Check sheet for the modelled part. Datum: model origin and axes. Units: mm. Face numbers are marked on the shaded views. A direction names the side the tool comes from. Give positions to 0.01 mm unless a question says otherwise; leave off trailing zeros. Order: outer loops, then holes, each group sorted by start corner. A loop starts at its lowest first (then second) coordinate and runs counter-clockwise, first axis right, second up.
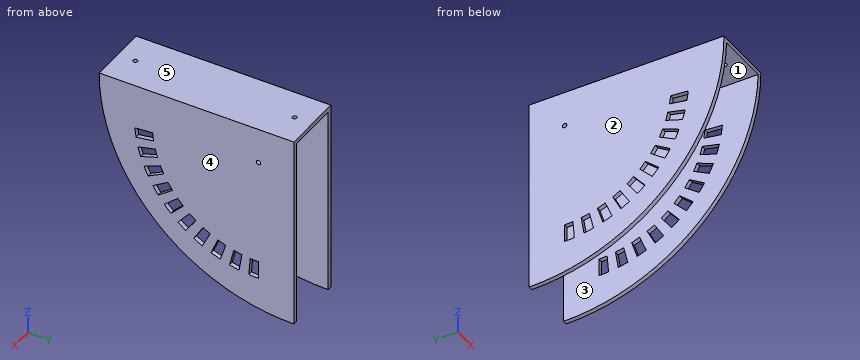
```python
from build123d import *

# Parameters (mm, degrees)
SKETCH1_W             = 5
SKETCH1_H             = 220
BOSS_EXTRUDE1_DEPTH   = 220
BOSS_EXTRUDE1_2_DEPTH = 220
SKETCH2_W             = 60
SKETCH2_H             = 220
BOSS_EXTRUDE2_DEPTH   = 5
CUT_EXTRUDE1_DEPTH    = 110
SKETCH7_R             = 2.5
CUT_EXTRUDE6_DEPTH    = 134
SKETCH9_R             = 2.5
CUT_EXTRUDE8_DEPTH    = 134


with BuildPart() as part:
    # Sketch1 → Boss-Extrude1 (new body)
    with BuildSketch(Plane.XY):
        with Locations((32.5, 0)):
            Rectangle(SKETCH1_W, SKETCH1_H)
    extrude(amount=BOSS_EXTRUDE1_DEPTH)



with BuildPart() as body_2:
    # Sketch1 → Boss-Extrude1 2 (new body)
    with BuildSketch(Plane.XY):
        with Locations((-32.5, 0)):
            Rectangle(SKETCH1_W, SKETCH1_H)
    extrude(amount=BOSS_EXTRUDE1_2_DEPTH)


with BuildPart() as part_1:
    add(part.part)

    add(body_2.part)  # Boss-Extrude2 merges body 2
    # Sketch2 → Boss-Extrude2 (add)
    with BuildSketch(Plane.XY.offset(220)):
        Rectangle(SKETCH2_W, SKETCH2_H)
    extrude(amount=-BOSS_EXTRUDE2_DEPTH)

    # Sketch3 → Cut-Extrude1 (cut)
    with BuildSketch(Plane.ZY.offset(35)):
        with BuildLine():
            Line((0, 110), (0, -110))
            Line((0, -110), (220, -110))
            ThreePointArc((220, -110), (64.436508139, -45.563491861), (0, 110))
        make_face()
    extrude(amount=-CUT_EXTRUDE1_DEPTH, mode=Mode.SUBTRACT)

    # Sketch7 → Cut-Extrude6 (cut)
    with BuildSketch(Plane(origin=(0, 0, 215), x_dir=(-1, 0, 0), z_dir=(0, 0, -1))):
        with Locations((0, 90)):
            Circle(SKETCH7_R)
        with Locations((0, -90)):
            Circle(SKETCH7_R)
    extrude(amount=-CUT_EXTRUDE6_DEPTH, mode=Mode.SUBTRACT)

    # Sketch9 → Cut-Extrude8 (cut)
    with BuildSketch(Plane.ZY.offset(35)):
        with BuildLine():
            ThreePointArc((60.369919952, 60.584908513), (60.092515651, 65.288822109), (60, 70))
            Line((60, 70), (40, 70))
            ThreePointArc((40, 70), (40.107934926, 64.503625794), (40.431573277, 59.015726598))
            Line((40.431573277, 59.015726598), (60.369919952, 60.584908513))
        make_face()
        with BuildLine():
            ThreePointArc((63.315609552, 41.986556337), (62.305766352, 46.589161358), (61.477399129, 51.227864195))
            Line((61.477399129, 51.227864195), (41.723632317, 48.099174894))
            ThreePointArc((41.723632317, 48.099174894), (42.690060744, 42.687354918), (43.868211144, 37.31764906))
            Line((43.868211144, 37.31764906), (63.315609552, 41.986556337))
        make_face()
        with BuildLine():
            ThreePointArc((69.134456099, 24.077988116), (67.417039689, 28.465953151), (65.873218045, 32.917960675))
            Line((65.873218045, 32.917960675), (46.852087719, 26.737620788))
            ThreePointArc((46.852087719, 26.737620788), (48.653212971, 21.543612009), (50.656865448, 16.424319469))
            Line((50.656865448, 16.424319469), (69.134456099, 24.077988116))
        make_face()
        with BuildLine():
            ThreePointArc((77.683180278, 7.300172234), (75.300479151, 11.36545102), (73.079217097, 15.521140031))
            Line((73.079217097, 15.521140031), (55.259086614, 6.441330036))
            ThreePointArc((55.259086614, 6.441330036), (57.85055901, 1.59302619), (60.63037699, -3.14979906))
            Line((60.63037699, -3.14979906), (77.683180278, 7.300172234))
        make_face()
        with BuildLine():
            ThreePointArc((88.751284128, -7.9337658), (85.761968294, -4.291273917), (82.917960675, -0.534230275))
            Line((82.917960675, -0.534230275), (66.737620788, -12.289935321))
            ThreePointArc((66.737620788, -12.289935321), (70.055629677, -16.673152903), (73.543164816, -20.922726766))
            Line((73.543164816, -20.922726766), (88.751284128, -7.9337658))
        make_face()
        with BuildLine():
            ThreePointArc((102.0662342, -21.248715872), (98.543910536, -18.118701132), (95.147186258, -14.852813742))
            Line((95.147186258, -14.852813742), (81.005050634, -28.994949366))
            ThreePointArc((81.005050634, -28.994949366), (84.967895625, -32.805151321), (89.077273234, -36.456835184))
            Line((89.077273234, -36.456835184), (102.0662342, -21.248715872))
        make_face()
        with BuildLine():
            ThreePointArc((117.300172234, -32.316819722), (113.331572038, -29.776353476), (109.465769725, -27.082039325))
            Line((109.465769725, -27.082039325), (97.710064679, -43.262379212))
            ThreePointArc((97.710064679, -43.262379212), (102.220167377, -46.405745722), (106.85020094, -49.36962301))
            Line((106.85020094, -49.36962301), (117.300172234, -32.316819722))
        make_face()
        with BuildLine():
            ThreePointArc((134.077988116, -40.865543901), (129.760831496, -38.977180859), (125.521140031, -36.920782903))
            Line((125.521140031, -36.920782903), (116.441330036, -54.740913386))
            ThreePointArc((116.441330036, -54.740913386), (121.387636745, -57.140044336), (126.424319469, -59.343134552))
            Line((126.424319469, -59.343134552), (134.077988116, -40.865543901))
        make_face()
        with BuildLine():
            ThreePointArc((151.986556337, -46.684390448), (147.427146016, -45.494628374), (142.917960675, -44.126781955))
            Line((142.917960675, -44.126781955), (136.737620788, -63.147912281))
            ThreePointArc((136.737620788, -63.147912281), (141.998337019, -64.743733104), (147.31764906, -66.131788856))
            Line((147.31764906, -66.131788856), (151.986556337, -46.684390448))
        make_face()
        with BuildLine():
            ThreePointArc((170.584908513, -49.630080048), (165.895512305, -49.168214835), (161.227864195, -48.522600871))
            Line((161.227864195, -48.522600871), (158.099174894, -68.276367683))
            ThreePointArc((158.099174894, -68.276367683), (163.544764356, -69.029583974), (169.015726598, -69.568426723))
            Line((169.015726598, -69.568426723), (170.584908513, -49.630080048))
        make_face()
        with Locations((180, 70)):
            Circle(SKETCH9_R)
    extrude(amount=-CUT_EXTRUDE8_DEPTH, mode=Mode.SUBTRACT)


solid = part_1.part
```
(1) Cross-section at A-A on z = 196.5. Enter the section's corners in (x, y), then the cut area to 3 significant figures.
Response values:
outline: (-35, -108.74) - (-30, -108.74) - (-30, 110) - (-35, 110) - close; (30, -108.74) - (35, -108.74) - (35, 110) - (30, 110) - close
area: 2,190 mm2
(2) Cross-section at D-D on z = 17. Enter the section's corners in (x, y), then the cut area to 3 significant figures.
Response values:
outline: (-35, 25.2) - (-30, 25.2) - (-30, 110) - (-35, 110) - close; (30, 25.2) - (35, 25.2) - (35, 110) - (30, 110) - close
area: 848 mm2
(3) Gauge pin test, flat ends, axial feed: pin 1 Ø1.5 at (x, y) = (9, -80.5) entering from -Z; pin 2 Ø4 at (x, z) = (33.5, 48.5) entering from -Y; pin 3 Ø4 at (x, y) = (0, 90) entering from +Z; pin 4 Ø4 at (x, z) = (-32, 52) entering from -Y. Record the tip position at first contact, or that the pin passes through.
Response values:
pin 1: stops at z = 215
pin 2: stops at y = -30.25
pin 3: passes through
pin 4: stops at y = -34.37
(4) Set-up check for the marked faces 1 and 2: record each of +Z, -Z, +X, -X, +Y, -Y from which the full face is reachable in a straight line by a thin tool's end or side.
Response values:
face 1: -Z, +Y, -Y
face 2: +Z, -Z, -X, +Y, -Y
(5) Cross-section at B-B on y = 11.5. Enter the section's corners in (x, z).
Response values:
outline: (-35, 23.28) - (-30, 23.28) - (-30, 65.19) - (-35, 65.19) - close; (-35, 75.23) - (-30, 75.23) - (-30, 215) - (30, 215) - (30, 75.23) - (35, 75.23) - (35, 220) - (-35, 220) - close; (30, 23.28) - (35, 23.28) - (35, 65.19) - (30, 65.19) - close
(6) Cross-section at C-C on x = 14.5. Enter the section's corners in (y, z).
Response values:
outline: (-110, 220) arc R220 ccw to (-109.94, 215) - (110, 215) - (110, 220) - close
(7) Release check for a two-part mould opening along X. For the marked faces 3, 4 and 5 record: released by +X, released by -X, zero draft, split by the parting line, or undercut.
Response values:
face 3: undercut
face 4: released by +X
face 5: zero draft
(8) Material ranges on L1, parallel to Y at x = 0, z = 217.3; L2, parallel to X at y = 12.5, z = 57; L3, parallel to Y at x = -31.4, z = 180, recorded low to high.
Response values:
L1: y = -109.98 to -92.5, -87.5 to 87.5, 92.5 to 110
L2: x = -35 to -30, 30 to 35
L3: y = -106.33 to 67.5, 72.5 to 110
